from build123d import *

# Parameters (mm, degrees)
BOSS_EXTRUDE1_DEPTH = 2330
SKETCH3_W           = 1100
SKETCH3_H           = 2030
CUT_EXTRUDE1_DEPTH  = 3000


with BuildPart() as part:
    # Sketch2 → Boss-Extrude1 (new body)
    with BuildSketch(Plane(origin=(0, 0, 0), x_dir=(1, 0, 0), z_dir=(0, 1, 0))):
        with BuildLine():
            Line((-6692.186143144, -5017.367964626), (-6692.186143144, -5267.367964626))
            Line((-6692.186143144, -5267.367964626), (-8092.186143144, -5267.367964626))
            Line((-8092.186143144, -5267.367964626), (-8092.186143144, -5030.09988938))
            ThreePointArc((-8092.186143144, -5030.09988938), (-7392.105105324, -5032.64483009), (-6692.186143144, -5017.367964626))
        make_face()
    extrude(amount=BOSS_EXTRUDE1_DEPTH)

    # Sketch3 → Cut-Extrude1 (cut)
    with BuildSketch(Plane.XY.offset(5267.367964626)):
        with Locations((-7392.186143144, 1165)):
            Rectangle(SKETCH3_W, SKETCH3_H)
    extrude(amount=-CUT_EXTRUDE1_DEPTH, mode=Mode.SUBTRACT)


solid = part.part
The listing builds one solid part. Answer for the finished solid, in the listing's coordinates (mm). A direction names the side the tool comes from. Coordinates: 2 decimals unless noted, no trailing zeros. Order: outer loops, then holes, each group sorted by start corner. A loop starts at its lowest first (then second) coordinate and runs counter-clockwise, first axis right, second up.
Q1. A cutting plane is placed at A-A, the plane y = 1263.5. Write down the section's boundary in (x, z), and give its area (3 significant figures).
Q2. A cutting plane is placed at B-B, the plane z = 5236. Write down the section's boundary in (x, y), and give its area (3 significant figures).
Q3. Consider line 1 (Y direction, x = -7615, z = 5236); line 2 (X direction, y = 1218, z = 5078.5); line 3 (X direction, y = 319, z = 5029). Determine where each line is inside the solid, lowest interval first.
Q4. A cutting plane is placed at C-C, the plane x = -7153.5. Write down the section's boundary in (y, z).
Q5. Given P1, Ø1.5, axis at x = -7262, z = 5161, coming from the -Y side, flat-ended and moving along its own axis, determine where the tip first touches the part or whether it passes through.
Q6. A cutting plane is placed at D-D, the plane x = -8003.5. Write down the section's boundary in (y, z), and give its area (3 significant figures).
Q7. For a pull along Y with two mould halves and no side action, classify faces 1 (the face through (-7382, 2330, 5141)), 2 (the face through (-7382, 0, 5141)), 3 (the face through (-8005, 1149, 5267.368)), 4 (the face through (-7942.186, 1151, 5151)) as pulls with the +Y half, pulls with the -Y half, needs draft (parallel to the pull), parting line crosses it, or undercut.
Q8. Which of the six approach directions +Z, -Z, +X, -X, +Y, -Y give full straight-line access (tool end or side, diameter ignored) to faces 5 (the face through (-8024.21, 1148.69, 5031.13)), 6 (the face through (-7400, 2180, 5146)), 7 (the face through (-6692.186, 1149, 5141))?
Answers follow:
1. outline: (-8092.19, 5030.1) arc R27500 cw to (-7942.19, 5032.15) - (-7942.19, 5267.37) - (-8092.19, 5267.37) - close; (-6842.19, 5022.14) arc R27500 cw to (-6692.19, 5017.37) - (-6692.19, 5267.37) - (-6842.19, 5267.37) - close
1. area: 72,600 mm2
2. outline: (-8092.19, 0) - (-6692.19, 0) - (-6692.19, 2330) - (-8092.19, 2330) - close; hole (-7942.19, 150) - (-6842.19, 150) - (-6842.19, 2180) - (-7942.19, 2180) - close
2. area: 1,030,000 mm2
3. line 1: y = 0 to 150, 2180 to 2330
3. line 2: x = -8092.19 to -7942.19, -6842.19 to -6692.19
3. line 3: x = -6842.19 to -6692.19
4. outline: (0, 5029.44) - (150, 5029.44) - (150, 5267.37) - (0, 5267.37) - close; (2180, 5029.44) - (2330, 5029.44) - (2330, 5267.37) - (2180, 5267.37) - close
5. P1: stops at y = 0
6. outline: (0, 5031.41) - (2330, 5031.41) - (2330, 5267.37) - (0, 5267.37) - close
6. area: 550,000 mm2
7. face 1: pulls with the +Y half
7. face 2: pulls with the -Y half
7. face 3: needs draft
7. face 4: undercut
8. face 5: -Z, +Y, -Y
8. face 6: +Z, -Z
8. face 7: +Z, -Z, +X, +Y, -Y
